```python
from build123d import *

# Parameters (mm, degrees)
F1_W     = 240
F1_H     = 38
F2_DEPTH = 8
F3_W     = 240
F3_H     = 35
F4_DEPTH = 1
F5_W     = 3
F5_H     = 3
F6_DEPTH = 3


with BuildPart() as f2:
    # F1 (on Top) → F2 (new body)
    with BuildSketch(Plane.XY):
        Rectangle(F1_W, F1_H)
    extrude(amount=F2_DEPTH)

    # F3 (on face) → F4 (cut)
    with BuildSketch(Plane.XY.offset(8)):
        with Locations((0, -1.5)):
            Rectangle(F3_W, F3_H)
    extrude(amount=-F4_DEPTH, mode=Mode.SUBTRACT)

    # F5 (on face) → F6 (join)
    with BuildSketch(Plane.XY.offset(8)):
        with Locations((118.5, 17.5)):
            Rectangle(F5_W, F5_H)
    extrude(amount=F6_DEPTH)


solid = f2.part
```
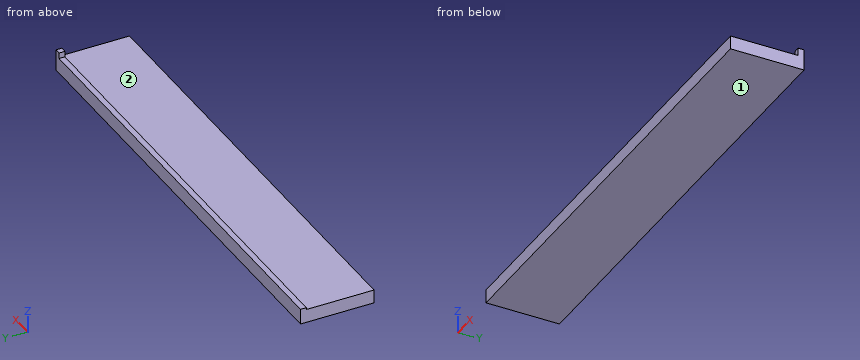
Geometry check sheet. Reference: the model listing, model coordinates, mm. Face numbers are marked on the shaded views. A direction names the side the tool comes from. Give positions to 0.01 mm unless a question says otherwise; leave off trailing zeros. Write each loop counter-clockwise with the first axis right and the second up, starting at its lowest first coordinate (ties: lowest second). Pieces come first, ordered by that corner, then holes. Notation, with made-up numbers: (-5.75, -28) - (21.25, -28) arc R11 cw to (21.25, -10) - close; hole circle Ø7 at (35, 33.25). An arc over 180 degrees is marked (long way). Use a Markdown table: item, result.
Q1. Section check B-B, the plane y = -5. Enter the section's corners in (x, z), then the cut area to 3 significant figures.
Computed:
| item | result |
|---|---|
| outline | (-120, 0) - (120, 0) - (120, 7) - (-120, 7) - close |
| area | 1,680 mm² |
Q2. Section check A-A, the plane x = 87.5. Enter the section's corners in (y, z), then the cut area to 3 significant figures.
Computed:
| item | result |
|---|---|
| outline | (-19, 0) - (19, 0) - (19, 8) - (16, 8) - (16, 7) - (-19, 7) - close |
| area | 269 mm² |
Q3. Go/stop test with flat-tipped pins: P1, Ø12, axis at x = -45.5, y = -12, coming from the +Z side; P2, Ø1.5, axis at x = -0.5, y = 17.5, coming from the +Z side; P3, Ø1.5, axis at y = 17, z = 9.5, coming from the -X side. Record where each tip stops, or that it passes through.
Computed:
| item | result |
|---|---|
| P1 | stops at z = 7 |
| P2 | stops at z = 8 |
| P3 | stops at x = 117 |
Q4. Set-up check for the marked faces 1 and 2: record each of +Z, -Z, +X, -X, +Y, -Y from which the full face is reachable in a straight line by a thin tool's end or side.
Computed:
| item | result |
|---|---|
| face 1 | -Z, +X, -X, +Y, -Y |
| face 2 | +Z, +X, -X, -Y |
Q5. Thickness scan on L1, parallel to Z at x = -22.5, y = -5; L2, parallel to Y at x = -108, z = 7.25; L3, parallel to Z at x = 43, y = 16.5. Record the ranges inside material, lowest first. Write a range as [from, to].
Computed:
| item | result |
|---|---|
| L1 | z = [0, 7] |
| L2 | y = [16, 19] |
| L3 | z = [0, 8] |
